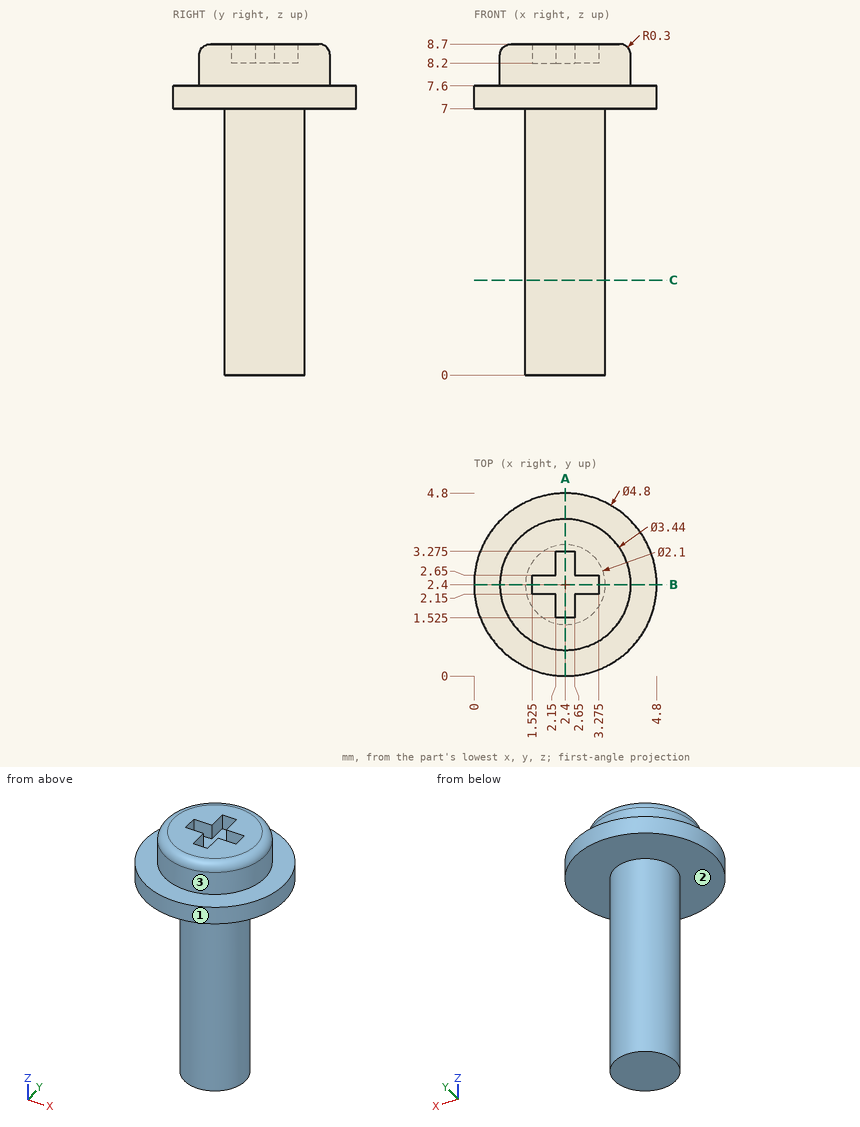
Answer from the drawing. Dimensions are ordinates in mm from the lowest x, y and z of the part. A direction names the side the tool comes from. Coordinates: 2 decimals unless noted, no trailing zeros. Order: outer loops, then holes, each group sorted by start corner. A loop starts at its lowest first (then second) coordinate and runs counter-clockwise, first axis right, second up. Notation, with made-up numbers: (66.5, 24.5) -> (116.5, 24.5) arc R22 ccw to (116.5, 57.5) -> close; hole circle Ø6 at (89.5, 52). An arc over 180 degrees is marked (long way). Answer as a JSON object with one key per item and string values.
1) Each of these flat-tipped pins is pushed along its axis until it touches: pin 1 (1 mm diameter, centred on y = 3.5, z = 2.5, fed in from -X); pin 2 (0.6 mm diameter, centred on y = 2.5, z = 8.5, fed in from +X); pin 3 (1 mm diameter, centred on y = 2, z = 3.5, fed in from -X). Where does it stop, or does it pass through?
Model answer:
{"pin 1": "stops at x = 1.54", "pin 2": "stops at x = 4.12", "pin 3": "stops at x = 1.35"}
2) A tool of negligible diameter and unlimited length cuts with its end or side. For the marked faces 1, 2 and 3, from which of +Z, -Z, +X, -X, +Y, -Y can it reach the whole face along a straight path? Write none if from no direction.
Model answer:
{"face 1": "+Z, -Z", "face 2": "-Z", "face 3": "+Z"}
3) Consider line 1 along Z through (x, y) = (3.2, 3.3); line 2 along Z through (x, y) = (4.1, 1.4); line 3 along X through (y, z) = (1.65, 2.5). Determine where each line is inside the solid, lowest interval first. Write a range as from..to.
Model answer:
{"line 1": "z = 7..8.7", "line 2": "z = 7..7.6", "line 3": "x = 1.67..3.13"}
4) A cutting plane is placed at A-A, the plane x = 2.4. Determine the outline of the cut face in (y, z) (3 decimals).
Model answer:
{"outline": "(0, 7) -> (1.35, 7) -> (1.35, 0) -> (3.45, 0) -> (3.45, 7) -> (4.8, 7) -> (4.8, 7.6) -> (4.12, 7.6) -> (4.12, 8.4) arc R0.3 ccw to (3.82, 8.7) -> (3.275, 8.7) -> (3.275, 8.2) -> (1.525, 8.2) -> (1.525, 8.7) -> (0.98, 8.7) arc R0.3 ccw to (0.68, 8.4) -> (0.68, 7.6) -> (0, 7.6) -> close"}
5) A cutting plane is placed at C-C, the plane z = 2.5. Determine the outline of the cut face in (x, y).
Model answer:
{"outline": "circle Ø2.1 at (2.4, 2.4)"}
